```python
from build123d import *

# Parameters (mm, degrees)
SKETCH1_R                = 0.8
ROOF_DEPTH               = 1
WALLS_START              = -4
SKETCH1_3_R              = 0.8
WALLS_DEPTH              = 4
SKETCH2_R                = 5.1
SCREW_HOLE_IN_ROOF_DEPTH = 18.146428369
SCREW_START              = 2.8
SKETCH2_3_R              = 7
SKETCH2_3_R_2            = 5.1
SCREW_HOLDER_DEPTH       = 2.8


with BuildPart() as part:
    # Sketch1 → Roof (new body)
    # profile 1 of 4: a face of its own
    with BuildSketch(Plane.XY):
        Polygon((-7.67766953, 10), (-10, 7.67766953), (-10, 2), (-10, -2), (-10, -7.67766953), (-7.67766953, -10), (7.67766953, -10), (10, -7.67766953), (10, -2), (10, 2), (10, 7.67766953), (7.67766953, 10), align=None)
        Polygon((-8.4, -7.01492783), (-8.4, 7.01492783), (-7.01492783, 8.4), (7.01492783, 8.4), (8.4, 7.01492783), (8.4, -7.01492783), (7.01492783, -8.4), (-7.01492783, -8.4), align=None, mode=Mode.SUBTRACT)
    # profile 2 of 4: a face of its own
    with BuildSketch(Plane.XY):
        Polygon((7.01492783, 8.4), (-7.01492783, 8.4), (-8.4, 7.01492783), (-8.4, -7.01492783), (-7.01492783, -8.4), (7.01492783, -8.4), (8.4, -7.01492783), (8.4, 7.01492783), align=None)
    # profile 3 of 4: a face of its own
    with BuildSketch(Plane.XY):
        with BuildLine():
            Line((-10, -2), (-10, 2))
            Line((-10, 2), (-11.000000224, 2))
            ThreePointArc((-11.000000224, 2), (-13.000000224, 0), (-11.000000224, -2))
            Line((-11.000000224, -2), (-10, -2))
        make_face()
        with Locations((-11.000000224, 0)):
            Circle(SKETCH1_R, mode=Mode.SUBTRACT)
    # profile 4 of 4: a face of its own
    with BuildSketch(Plane.XY):
        with BuildLine():
            Line((11, 2), (10, 2))
            Line((10, 2), (10, -2))
            Line((10, -2), (11, -2))
            ThreePointArc((11, -2), (13, 0), (11, 2))
        make_face()
        with Locations((11, 0)):
            Circle(SKETCH1_R, mode=Mode.SUBTRACT)
    extrude(amount=ROOF_DEPTH)

    # Sketch1_3 → Walls (add)
    # profile 1 of 3: a face of its own
    with BuildSketch(Plane.XY.offset(WALLS_START)):
        Polygon((-7.67766953, 10), (-10, 7.67766953), (-10, 2), (-10, -2), (-10, -7.67766953), (-7.67766953, -10), (7.67766953, -10), (10, -7.67766953), (10, -2), (10, 2), (10, 7.67766953), (7.67766953, 10), align=None)
        Polygon((-8.4, -7.01492783), (-8.4, 7.01492783), (-7.01492783, 8.4), (7.01492783, 8.4), (8.4, 7.01492783), (8.4, -7.01492783), (7.01492783, -8.4), (-7.01492783, -8.4), align=None, mode=Mode.SUBTRACT)
    # profile 2 of 3: a face of its own
    with BuildSketch(Plane.XY.offset(WALLS_START)):
        with BuildLine():
            Line((11, 2), (10, 2))
            Line((10, 2), (10, -2))
            Line((10, -2), (11, -2))
            ThreePointArc((11, -2), (13, 0), (11, 2))
        make_face()
        with Locations((11, 0)):
            Circle(SKETCH1_3_R, mode=Mode.SUBTRACT)
    # profile 3 of 3: a face of its own
    with BuildSketch(Plane.XY.offset(WALLS_START)):
        with BuildLine():
            Line((-10, -2), (-10, 2))
            Line((-10, 2), (-11.000000224, 2))
            ThreePointArc((-11.000000224, 2), (-13.000000224, 0), (-11.000000224, -2))
            Line((-11.000000224, -2), (-10, -2))
        make_face()
        with Locations((-11.000000224, 0)):
            Circle(SKETCH1_3_R, mode=Mode.SUBTRACT)
    extrude(amount=WALLS_DEPTH)

    # Sketch2 → Screw hole in roof (cut, through all)
    with BuildSketch(Plane.XY.offset(1)):
        Circle(SKETCH2_R)
    extrude(amount=-SCREW_HOLE_IN_ROOF_DEPTH, mode=Mode.SUBTRACT)

    # Sketch2_3 → Screw holder (add)
    with BuildSketch(Plane.XY.offset(1).offset(SCREW_START)):
        Circle(SKETCH2_3_R)
        Circle(SKETCH2_3_R_2, mode=Mode.SUBTRACT)
    extrude(amount=-SCREW_HOLDER_DEPTH)


solid = part.part
```
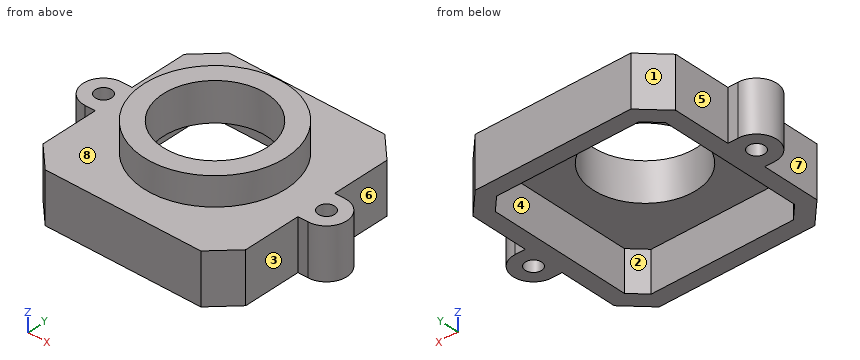
The listing builds one solid part. Answer for the finished solid, in the listing's coordinates (mm). Face numbers are marked on the shaded views. A direction names the side the tool comes from. Coordinates: 2 decimals unless noted, no trailing zeros. Write each loop counter-clockwise with the first axis right and the second up, starting at its lowest first coordinate (ties: lowest second). Pieces come first, ordered by that corner, then holes.
Q1. Section C-C, the plane z = -3 is taken. Write down the section's boundary in (x, y).
Returned:
outline: (-11, -2) - (-10, -2) - (-10, -7.68) - (-7.68, -10) - (7.68, -10) - (10, -7.68) - (10, -2) - (11, -2) arc R2 ccw to (11, 2) - (10, 2) - (10, 7.68) - (7.68, 10) - (-7.68, 10) - (-10, 7.68) - (-10, 2) - (-11, 2) arc R2 ccw to start; hole circle Ø1.6 at (-11, 0); hole (-8.4, -7.01) - (-7.01, -8.4) - (7.01, -8.4) - (8.4, -7.01) - (8.4, 7.01) - (7.01, 8.4) - (-7.01, 8.4) - (-8.4, 7.01) - close; hole circle Ø1.6 at (11, 0)
Q2. Section A-A, the plane y = 0 is taken. Write down the section's boundary in (x, z).
Returned:
outline: (-13, -4) - (-11.8, -4) - (-11.8, 1) - (-13, 1) - close; (-10.2, -4) - (-8.4, -4) - (-8.4, 0) - (-5.1, 0) - (-5.1, 3.8) - (-7, 3.8) - (-7, 1) - (-10.2, 1) - close; (5.1, 0) - (8.4, 0) - (8.4, -4) - (10.2, -4) - (10.2, 1) - (7, 1) - (7, 3.8) - (5.1, 3.8) - close; (11.8, -4) - (13, -4) - (13, 1) - (11.8, 1) - close
Q3. Which of the six approach directions +Z, -Z, +X, -X, +Y, -Y give full straight-line access (tool end or side, diameter ignored) to the marked faces 4, 5, 6, 7 and 8?
Returned:
face 4: -Z
face 5: +Z, -Z, -X, +Y
face 6: +Z, -Z, +X, +Y
face 7: +Z, -Z, -X, -Y
face 8: +Z
Q4. Given P1, Ø0.8, axis at x = -10.5, z = -2.5, coming from the +Y side; P2, Ø1, axis at y = 5, z = 2, coming from the -X side; P3, Ø0.5, axis at x = -10.5, z = -1, coming from the -Y side, each flat-ended and moving along its own axis, determine where each tip first touches the part or whether it passes through.
Returned:
P1: stops at y = 2
P2: stops at x = -5.36
P3: stops at y = -2
Q5. Find the intervals of material crossed by line 1 along Y through (x, z) = (-3, -1.25); line 2 along Y through (x, z) = (11, -2.5); line 3 along X through (y, z) = (-7.25, 0.5), in increasing order.
Returned:
line 1: y = -10 to -8.4, 8.4 to 10
line 2: y = -2 to -0.8, 0.8 to 2
line 3: x = -10 to 10
Q6. Section B-B, the plane x = 0 is taken. Write down the section's boundary in (y, z), then the cut area to 3 significant figures.
Returned:
outline: (-10, -4) - (-8.4, -4) - (-8.4, 0) - (-5.1, 0) - (-5.1, 3.8) - (-7, 3.8) - (-7, 1) - (-10, 1) - close; (5.1, 0) - (8.4, 0) - (8.4, -4) - (10, -4) - (10, 1) - (7, 1) - (7, 3.8) - (5.1, 3.8) - close
area: 33.2 mm2
Q7. Section D-D, the plane y = 4.5 is taken. Write down the section's boundary in (x, z), then the cut area to 3 significant figures.
Returned:
outline: (-10, -4) - (-8.4, -4) - (-8.4, 0) - (-2.4, 0) - (-2.4, 3.8) - (-5.36, 3.8) - (-5.36, 1) - (-10, 1) - close; (2.4, 0) - (8.4, 0) - (8.4, -4) - (10, -4) - (10, 1) - (5.36, 1) - (5.36, 3.8) - (2.4, 3.8) - close
area: 44.6 mm2
Q8. The mould has two halves that part along Y. Classify the marked faces 1, 2 and 3: released by +Y, released by -Y, zero draft, split by the parting line, or undercut.
Returned:
face 1: released by +Y
face 2: undercut
face 3: zero draft
